Verification items for the finished model (mm, model axes). Give positions to 0.01 mm unless a question says otherwise; leave off trailing zeros. Order: outer loops, then holes, each group sorted by start corner. A loop starts at its lowest first (then second) coordinate and runs counter-clockwise, first axis right, second up. Notation, with made-up numbers: (2, 36.25) - (7, 36.25) arc R36 ccw to (7, 70.25) - close; hole circle Ø10 at (-11.75, -2). An arc over 180 degrees is marked (long way). Answer as a JSON object with one key per item and string values.
```python
from build123d import *

# Parameters (mm, degrees)
CYLINDER_R     = 1.5
CYLINDER_DEPTH = 10
BOX008_W       = 7
BOX008_H       = 7
BOX008_DEPTH   = 4.5


with BuildPart() as hole:
    # Cylinder → Cylinder (new body)
    with BuildSketch(Plane.XY):
        Circle(CYLINDER_R)
    extrude(amount=CYLINDER_DEPTH)


with BuildPart() as stand_hole_cut:
    # Box008 → Box008 (new body)
    with BuildSketch(Plane(origin=(-3.5, -3.5, 0), x_dir=(1, 0, 0), z_dir=(0, 0, 1))):
        with Locations((3.5, 3.5)):
            Rectangle(BOX008_W, BOX008_H)
    extrude(amount=BOX008_DEPTH)

    # Cut003002: cut hole
    add(hole.part, mode=Mode.SUBTRACT)


solid = stand_hole_cut.part
```
(1) Material ranges on line 1 along X through (y, z) = (0, 2.45); line 2 along X through (y, z) = (-0.75, 3), recorded low to high. Write a range as [from, to].
Computed values:
{"line 1": "x = [-3.5, -1.5], [1.5, 3.5]", "line 2": "x = [-3.5, -1.3], [1.3, 3.5]"}
(2) Section check A-A (y = 0). Record the cut outline in (x, z).
Computed values:
{"outline": "(-3.5, 0) - (-1.5, 0) - (-1.5, 4.5) - (-3.5, 4.5) - close; (1.5, 0) - (3.5, 0) - (3.5, 4.5) - (1.5, 4.5) - close"}
(3) Release check for a two-part mould opening along X. For faces 1 (the cylindrical face through (-1.5, 0.07, 2.22)), 2 (the flat face through (-3.5, 0, 2)), 3 (the flat face through (0, 3.5, 2)), 4 (the flat face through (3.5, 0, 2)) record: pulls with the +X half, pulls with the -X half, needs draft (parallel to the pull), parting line crosses it, or undercut.
Computed values:
{"face 1": "undercut", "face 2": "pulls with the -X half", "face 3": "needs draft", "face 4": "pulls with the +X half"}
(4) Gauge pin test, flat end, axial feed: pin 1 Ø1.8 at (x, y) = (0, 0) entering from -Z. Record the tip position at first contact, or that the pin passes through.
Computed values:
{"pin 1": "passes through"}
(5) Section check C-C (z = 0.55). Record the cut outline in (x, y).
Computed values:
{"outline": "(-3.5, -3.5) - (3.5, -3.5) - (3.5, 3.5) - (-3.5, 3.5) - close; hole circle Ø3 at (0, 0)"}
